Work out the finished part from the listing and answer in its coordinate system (mm). Face numbers are marked on the shaded views. A direction names the side the tool comes from. Coordinates: 2 decimals unless noted, no trailing zeros. Write each loop counter-clockwise with the first axis right and the second up, starting at its lowest first coordinate (ties: lowest second). Pieces come first, ordered by that corner, then holes. Notation, with made-up numbers: M 8,69 L 52,69 A14 cw 52,83 Z; hole C -2,18 d4. An arc over 180 degrees is marked long. Answer as CSV lines item,"result". Start each with the question number.
(1) A cutting plane is placed at A-A on z = 35. Give the vertices of the cut face in (x, y).
(2) The mould has two halves that part along Y. Classify the marked faces 1, 2 and 3: released by +Y, released by -Y, zero draft, split by the parting line, or undercut.
(3) Find the intervals of material crossed by L1, parallel to Z at x = -33.5, y = -20.5; L2, parallel to Z at x = 59.5, y = 51; L3, parallel to Y at x = -38.5, z = 32.5, in increasing order. Write a range as [from, to].
(4) For the marked faces 4 and 5, determine the directions among +Z, -Z, +X, -X, +Y, -Y from which every point of the face is accessible in a straight line to the end or side of a thin tool.
(5) Flat-ended cylindrical pins translate along their axes: P1, Ø8, axis at x = 13, z = 36.5, coming from the -Y side; P2, Ø4, axis at x = 29.43, y = -27.09, coming from the -Z side; P3, Ø4, axis at x = 46.5, y = 30, coming from the -Z side. Find the tip coordinate at first contact, or state that the pin passes through.
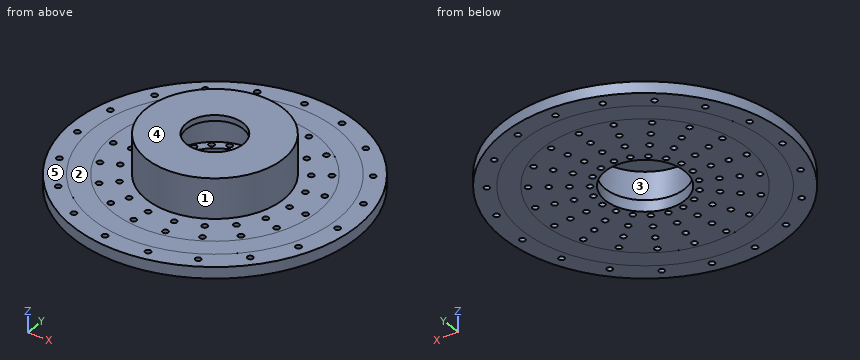
from build123d import *

# Parameters (mm, degrees)
SKETCH1_R                = 125
SKETCH1_R_2              = 35
SKETCH1_R_3              = 2.5
BOSS_EXTRUDE1_DEPTH      = 10
SKETCH2_R                = 60.29579013
SKETCH2_R_2              = 43.588302538
BOSS_EXTRUDE2_DEPTH      = 30
SKETCH3_R                = 60.29579013
BOSS_EXTRUDE3_DEPTH      = 5
SKETCH4_R                = 25
CUT_EXTRUDE2_DEPTH       = 47.5
SKETCH5_R                = 107.79610162
SKETCH5_R_2              = 90.298614491
BOSS_EXTRUDE4_DEPTH      = 10.001
BOSS_EXTRUDE4_DEPTH_BACK = 0.001


with BuildPart() as part:
    # Sketch1 → Boss-Extrude1 (new body)
    with BuildSketch(Plane.XY):
        Circle(SKETCH1_R)
        Circle(SKETCH1_R_2, mode=Mode.SUBTRACT)
        with Locations((0, 40)):
            Circle(SKETCH1_R_3, mode=Mode.SUBTRACT)
        with Locations((0, 55)):
            Circle(SKETCH1_R_3, mode=Mode.SUBTRACT)
        with Locations((0, 70)):
            Circle(SKETCH1_R_3, mode=Mode.SUBTRACT)
        with Locations((0, 85)):
            Circle(SKETCH1_R_3, mode=Mode.SUBTRACT)
        with Locations((0, 100)):
            Circle(SKETCH1_R_3, mode=Mode.SUBTRACT)
        with Locations((0, 115)):
            Circle(SKETCH1_R_3, mode=Mode.SUBTRACT)
        with Locations((37.340438959, 108.768982796)):
            Circle(SKETCH1_R_3, mode=Mode.SUBTRACT)
        with Locations((32.46994692, 94.58172417)):
            Circle(SKETCH1_R_3, mode=Mode.SUBTRACT)
        with Locations((27.599454882, 80.394465545)):
            Circle(SKETCH1_R_3, mode=Mode.SUBTRACT)
        with Locations((22.728962844, 66.207206919)):
            Circle(SKETCH1_R_3, mode=Mode.SUBTRACT)
        with Locations((17.858470806, 52.019948294)):
            Circle(SKETCH1_R_3, mode=Mode.SUBTRACT)
        with Locations((12.987978768, 37.832689668)):
            Circle(SKETCH1_R_3, mode=Mode.SUBTRACT)
        with Locations((70.634461959, 90.751158581)):
            Circle(SKETCH1_R_3, mode=Mode.SUBTRACT)
        with Locations((61.421271269, 78.91405094)):
            Circle(SKETCH1_R_3, mode=Mode.SUBTRACT)
        with Locations((52.208080579, 67.076943299)):
            Circle(SKETCH1_R_3, mode=Mode.SUBTRACT)
        with Locations((42.994889888, 55.239835658)):
            Circle(SKETCH1_R_3, mode=Mode.SUBTRACT)
        with Locations((33.781699198, 43.402728017)):
            Circle(SKETCH1_R_3, mode=Mode.SUBTRACT)
        with Locations((24.568508508, 31.565620376)):
            Circle(SKETCH1_R_3, mode=Mode.SUBTRACT)
        with Locations((96.274145, 62.899038184)):
            Circle(SKETCH1_R_3, mode=Mode.SUBTRACT)
        with Locations((83.716647826, 54.694815812)):
            Circle(SKETCH1_R_3, mode=Mode.SUBTRACT)
        with Locations((71.159150652, 46.49059344)):
            Circle(SKETCH1_R_3, mode=Mode.SUBTRACT)
        with Locations((58.601653478, 38.286371069)):
            Circle(SKETCH1_R_3, mode=Mode.SUBTRACT)
        with Locations((46.044156304, 30.082148697)):
            Circle(SKETCH1_R_3, mode=Mode.SUBTRACT)
        with Locations((33.486659131, 21.877926325)):
            Circle(SKETCH1_R_3, mode=Mode.SUBTRACT)
        with Locations((111.481030583, 28.230831021)):
            Circle(SKETCH1_R_3, mode=Mode.SUBTRACT)
        with Locations((96.940026594, 24.548548714)):
            Circle(SKETCH1_R_3, mode=Mode.SUBTRACT)
        with Locations((82.399022605, 20.866266407)):
            Circle(SKETCH1_R_3, mode=Mode.SUBTRACT)
        with Locations((67.858018616, 17.1839841)):
            Circle(SKETCH1_R_3, mode=Mode.SUBTRACT)
        with Locations((53.317014627, 13.501701793)):
            Circle(SKETCH1_R_3, mode=Mode.SUBTRACT)
        with Locations((38.776010638, 9.819419486)):
            Circle(SKETCH1_R_3, mode=Mode.SUBTRACT)
        with Locations((114.607216696, -9.496624729)):
            Circle(SKETCH1_R_3, mode=Mode.SUBTRACT)
        with Locations((99.658449301, -8.257934547)):
            Circle(SKETCH1_R_3, mode=Mode.SUBTRACT)
        with Locations((84.709681906, -7.019244365)):
            Circle(SKETCH1_R_3, mode=Mode.SUBTRACT)
        with Locations((69.76091451, -5.780554183)):
            Circle(SKETCH1_R_3, mode=Mode.SUBTRACT)
        with Locations((54.812147115, -4.541864001)):
            Circle(SKETCH1_R_3, mode=Mode.SUBTRACT)
        with Locations((39.86337972, -3.303173819)):
            Circle(SKETCH1_R_3, mode=Mode.SUBTRACT)
        with Locations((105.313932565, -46.194973835)):
            Circle(SKETCH1_R_3, mode=Mode.SUBTRACT)
        with Locations((91.577332666, -40.169542465)):
            Circle(SKETCH1_R_3, mode=Mode.SUBTRACT)
        with Locations((77.840732766, -34.144111095)):
            Circle(SKETCH1_R_3, mode=Mode.SUBTRACT)
        with Locations((64.104132866, -28.118679726)):
            Circle(SKETCH1_R_3, mode=Mode.SUBTRACT)
        with Locations((50.367532966, -22.093248356)):
            Circle(SKETCH1_R_3, mode=Mode.SUBTRACT)
        with Locations((36.630933066, -16.067816986)):
            Circle(SKETCH1_R_3, mode=Mode.SUBTRACT)
        with Locations((84.608249727, -77.887380737)):
            Circle(SKETCH1_R_3, mode=Mode.SUBTRACT)
        with Locations((73.572391067, -67.728157163)):
            Circle(SKETCH1_R_3, mode=Mode.SUBTRACT)
        with Locations((62.536532407, -57.568933588)):
            Circle(SKETCH1_R_3, mode=Mode.SUBTRACT)
        with Locations((51.500673747, -47.409710014)):
            Circle(SKETCH1_R_3, mode=Mode.SUBTRACT)
        with Locations((40.464815087, -37.250486439)):
            Circle(SKETCH1_R_3, mode=Mode.SUBTRACT)
        with Locations((29.428956427, -27.091262865)):
            Circle(SKETCH1_R_3, mode=Mode.SUBTRACT)
        with Locations((54.733950199, -101.139481389)):
            Circle(SKETCH1_R_3, mode=Mode.SUBTRACT)
        with Locations((47.594739304, -87.947375121)):
            Circle(SKETCH1_R_3, mode=Mode.SUBTRACT)
        with Locations((40.455528408, -74.755268853)):
            Circle(SKETCH1_R_3, mode=Mode.SUBTRACT)
        with Locations((33.316317513, -61.563162584)):
            Circle(SKETCH1_R_3, mode=Mode.SUBTRACT)
        with Locations((26.177106617, -48.371056316)):
            Circle(SKETCH1_R_3, mode=Mode.SUBTRACT)
        with Locations((19.037895722, -35.178950048)):
            Circle(SKETCH1_R_3, mode=Mode.SUBTRACT)
        with Locations((18.928377882, -113.431549891)):
            Circle(SKETCH1_R_3, mode=Mode.SUBTRACT)
        with Locations((16.459459028, -98.63613034)):
            Circle(SKETCH1_R_3, mode=Mode.SUBTRACT)
        with Locations((13.990540174, -83.840710789)):
            Circle(SKETCH1_R_3, mode=Mode.SUBTRACT)
        with Locations((11.52162132, -69.045291238)):
            Circle(SKETCH1_R_3, mode=Mode.SUBTRACT)
        with Locations((9.052702465, -54.249871687)):
            Circle(SKETCH1_R_3, mode=Mode.SUBTRACT)
        with Locations((6.583783611, -39.454452136)):
            Circle(SKETCH1_R_3, mode=Mode.SUBTRACT)
        with Locations((-18.928377882, -113.431549891)):
            Circle(SKETCH1_R_3, mode=Mode.SUBTRACT)
        with Locations((-16.459459028, -98.63613034)):
            Circle(SKETCH1_R_3, mode=Mode.SUBTRACT)
        with Locations((-13.990540174, -83.840710789)):
            Circle(SKETCH1_R_3, mode=Mode.SUBTRACT)
        with Locations((-11.52162132, -69.045291238)):
            Circle(SKETCH1_R_3, mode=Mode.SUBTRACT)
        with Locations((-9.052702465, -54.249871687)):
            Circle(SKETCH1_R_3, mode=Mode.SUBTRACT)
        with Locations((-6.583783611, -39.454452136)):
            Circle(SKETCH1_R_3, mode=Mode.SUBTRACT)
        with Locations((-54.733950199, -101.139481389)):
            Circle(SKETCH1_R_3, mode=Mode.SUBTRACT)
        with Locations((-47.594739304, -87.947375121)):
            Circle(SKETCH1_R_3, mode=Mode.SUBTRACT)
        with Locations((-40.455528408, -74.755268853)):
            Circle(SKETCH1_R_3, mode=Mode.SUBTRACT)
        with Locations((-33.316317513, -61.563162584)):
            Circle(SKETCH1_R_3, mode=Mode.SUBTRACT)
        with Locations((-26.177106617, -48.371056316)):
            Circle(SKETCH1_R_3, mode=Mode.SUBTRACT)
        with Locations((-19.037895721, -35.178950048)):
            Circle(SKETCH1_R_3, mode=Mode.SUBTRACT)
        with Locations((-84.608249727, -77.887380737)):
            Circle(SKETCH1_R_3, mode=Mode.SUBTRACT)
        with Locations((-73.572391067, -67.728157163)):
            Circle(SKETCH1_R_3, mode=Mode.SUBTRACT)
        with Locations((-62.536532407, -57.568933588)):
            Circle(SKETCH1_R_3, mode=Mode.SUBTRACT)
        with Locations((-51.500673747, -47.409710014)):
            Circle(SKETCH1_R_3, mode=Mode.SUBTRACT)
        with Locations((-40.464815087, -37.250486439)):
            Circle(SKETCH1_R_3, mode=Mode.SUBTRACT)
        with Locations((-29.428956427, -27.091262865)):
            Circle(SKETCH1_R_3, mode=Mode.SUBTRACT)
        with Locations((-105.313932565, -46.194973835)):
            Circle(SKETCH1_R_3, mode=Mode.SUBTRACT)
        with Locations((-91.577332665, -40.169542465)):
            Circle(SKETCH1_R_3, mode=Mode.SUBTRACT)
        with Locations((-77.840732766, -34.144111096)):
            Circle(SKETCH1_R_3, mode=Mode.SUBTRACT)
        with Locations((-64.104132866, -28.118679726)):
            Circle(SKETCH1_R_3, mode=Mode.SUBTRACT)
        with Locations((-50.367532966, -22.093248356)):
            Circle(SKETCH1_R_3, mode=Mode.SUBTRACT)
        with Locations((-36.630933066, -16.067816986)):
            Circle(SKETCH1_R_3, mode=Mode.SUBTRACT)
        with Locations((-114.607216696, -9.496624729)):
            Circle(SKETCH1_R_3, mode=Mode.SUBTRACT)
        with Locations((-99.658449301, -8.257934547)):
            Circle(SKETCH1_R_3, mode=Mode.SUBTRACT)
        with Locations((-84.709681906, -7.019244365)):
            Circle(SKETCH1_R_3, mode=Mode.SUBTRACT)
        with Locations((-69.76091451, -5.780554183)):
            Circle(SKETCH1_R_3, mode=Mode.SUBTRACT)
        with Locations((-54.812147115, -4.541864001)):
            Circle(SKETCH1_R_3, mode=Mode.SUBTRACT)
        with Locations((-39.86337972, -3.303173819)):
            Circle(SKETCH1_R_3, mode=Mode.SUBTRACT)
        with Locations((-111.481030583, 28.230831021)):
            Circle(SKETCH1_R_3, mode=Mode.SUBTRACT)
        with Locations((-96.940026594, 24.548548714)):
            Circle(SKETCH1_R_3, mode=Mode.SUBTRACT)
        with Locations((-82.399022605, 20.866266407)):
            Circle(SKETCH1_R_3, mode=Mode.SUBTRACT)
        with Locations((-67.858018616, 17.1839841)):
            Circle(SKETCH1_R_3, mode=Mode.SUBTRACT)
        with Locations((-53.317014627, 13.501701793)):
            Circle(SKETCH1_R_3, mode=Mode.SUBTRACT)
        with Locations((-38.776010638, 9.819419486)):
            Circle(SKETCH1_R_3, mode=Mode.SUBTRACT)
        with Locations((-96.274145, 62.899038184)):
            Circle(SKETCH1_R_3, mode=Mode.SUBTRACT)
        with Locations((-83.716647826, 54.694815812)):
            Circle(SKETCH1_R_3, mode=Mode.SUBTRACT)
        with Locations((-71.159150652, 46.49059344)):
            Circle(SKETCH1_R_3, mode=Mode.SUBTRACT)
        with Locations((-58.601653478, 38.286371069)):
            Circle(SKETCH1_R_3, mode=Mode.SUBTRACT)
        with Locations((-46.044156304, 30.082148697)):
            Circle(SKETCH1_R_3, mode=Mode.SUBTRACT)
        with Locations((-33.48665913, 21.877926325)):
            Circle(SKETCH1_R_3, mode=Mode.SUBTRACT)
        with Locations((-70.634461959, 90.751158581)):
            Circle(SKETCH1_R_3, mode=Mode.SUBTRACT)
        with Locations((-61.421271269, 78.91405094)):
            Circle(SKETCH1_R_3, mode=Mode.SUBTRACT)
        with Locations((-52.208080579, 67.076943299)):
            Circle(SKETCH1_R_3, mode=Mode.SUBTRACT)
        with Locations((-42.994889888, 55.239835658)):
            Circle(SKETCH1_R_3, mode=Mode.SUBTRACT)
        with Locations((-33.781699198, 43.402728017)):
            Circle(SKETCH1_R_3, mode=Mode.SUBTRACT)
        with Locations((-24.568508508, 31.565620376)):
            Circle(SKETCH1_R_3, mode=Mode.SUBTRACT)
        with Locations((-37.340438959, 108.768982796)):
            Circle(SKETCH1_R_3, mode=Mode.SUBTRACT)
        with Locations((-32.46994692, 94.58172417)):
            Circle(SKETCH1_R_3, mode=Mode.SUBTRACT)
        with Locations((-27.599454882, 80.394465545)):
            Circle(SKETCH1_R_3, mode=Mode.SUBTRACT)
        with Locations((-22.728962844, 66.207206919)):
            Circle(SKETCH1_R_3, mode=Mode.SUBTRACT)
        with Locations((-17.858470806, 52.019948294)):
            Circle(SKETCH1_R_3, mode=Mode.SUBTRACT)
        with Locations((-12.987978768, 37.832689668)):
            Circle(SKETCH1_R_3, mode=Mode.SUBTRACT)
    extrude(amount=BOSS_EXTRUDE1_DEPTH)

    # Sketch2 → Boss-Extrude2 (add)
    with BuildSketch(Plane.XY.offset(10)):
        Circle(SKETCH2_R)
        Circle(SKETCH2_R_2, mode=Mode.SUBTRACT)
    extrude(amount=BOSS_EXTRUDE2_DEPTH)

    # Sketch3 → Boss-Extrude3 (add)
    with BuildSketch(Plane.XY.offset(40)):
        Circle(SKETCH3_R)
    extrude(amount=BOSS_EXTRUDE3_DEPTH)

    # Sketch4 → Cut-Extrude2 (cut, symmetric)
    with BuildSketch(Plane(origin=(0, 0, 40), x_dir=(-1, 0, 0), z_dir=(0, 0, -1))):
        Circle(SKETCH4_R)
    extrude(amount=CUT_EXTRUDE2_DEPTH, both=True, mode=Mode.SUBTRACT)

    # Sketch5 → Boss-Extrude4 (add, two sides)
    with BuildSketch(Plane.XY) as boss_extrude4_sk:
        Circle(SKETCH5_R)
        Circle(SKETCH5_R_2, mode=Mode.SUBTRACT)
    extrude(amount=BOSS_EXTRUDE4_DEPTH)
    extrude(boss_extrude4_sk.sketch, amount=-BOSS_EXTRUDE4_DEPTH_BACK)


solid = part.part
Here are the results:
1,outline,"C 0,0 d120.59; hole C 0,0 d87.18"
2,face 1,"split by the parting line"
2,face 2,"zero draft"
2,face 3,"undercut"
3,L1,"z = [0, 10], [40, 45]"
3,L2,"z = [0, 10]"
3,L3,"y = [-46.4, -20.44], [20.44, 46.4]"
4,face 4,"+Z, +X, -X, +Y, -Y"
4,face 5,"+Z"
5,P1,"stops at y = -59.62"
5,P2,"stops at z = 40"
5,P3,"stops at z = 10"
